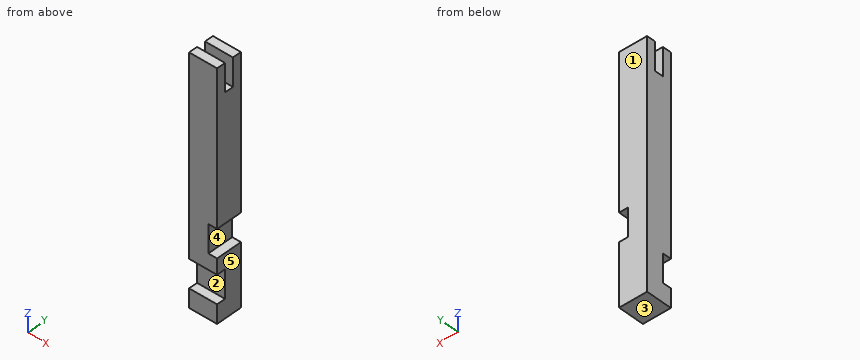
from build123d import *

# Parameters (mm, degrees)
F0_W     = 114.3
F0_H     = 106.68
F1_DEPTH = 990.6
F2_W     = 114.3
F2_H     = 35.56
F3_DEPTH = 114.3
F4_W     = 114.3
F4_H     = 114.3
F5_DEPTH = 35.56
F6_W     = 106.68
F6_H     = 114.3
F7_DEPTH = 35.56


with BuildPart() as f1:
    # F0 (on Top) → F1 (new body)
    with BuildSketch(Plane.XY):
        Rectangle(F0_W, F0_H)
    extrude(amount=F1_DEPTH)

    # F2 (on face) → F3 (cut)
    with BuildSketch(Plane.XY.offset(990.6)):
        Rectangle(F2_W, F2_H)
    extrude(amount=-F3_DEPTH, mode=Mode.SUBTRACT)

    # F4 (on face) → F5 (cut)
    with BuildSketch(Plane.XZ.offset(53.34)):
        with Locations((0, 133.35)):
            Rectangle(F4_W, F4_H)
    extrude(amount=-F5_DEPTH, mode=Mode.SUBTRACT)

    # F6 (on face) → F7 (cut)
    with BuildSketch(Plane.YZ.offset(57.15)):
        with Locations((0, 311.15)):
            Rectangle(F6_W, F6_H)
    extrude(amount=-F7_DEPTH, mode=Mode.SUBTRACT)


solid = f1.part
Check sheet for the modelled part. Datum: model origin and axes. Units: mm. Face numbers are marked on the shaded views. A direction names the side the tool comes from. Round coordinates to 2 decimals unless told otherwise and drop trailing zeros. Order: outer loops, then holes, each group sorted by start corner. A loop starts at its lowest first (then second) coordinate and runs counter-clockwise, first axis right, second up.
(1) Draft check along Z on the marked faces 3, 4 and 5. Enter one of: pulls with the +Z half, pulls with the -Z half, needs draft (parallel to the pull), parting line crosses it, or undercut.
(2) Access from +Z, -Z, +X, -X, +Y, -Y to the whole of each face (thin tool, end or side, straight path). Record for the marked faces 1 and 2.
(3) Cross-section at B-B, the plane y = -37.5. Enter the section's corners in (x, z), and give its area (3 significant figures).
(4) Cross-section at A-A, the plane z = 912. Enter the section's corners in (x, y), and give its area (3 significant figures).
(5) Cross-section at C-C, the plane y = 8. Enter the section's corners in (x, z).
(6) Cross-section at D-D, the plane x = 0. Enter the section's corners in (y, z), and give its area (3 significant figures).
(7) Scan lines: probe 1 along Z at (x, y) = (47, -44); probe 2 along Z at (x, y) = (48, -11.5); probe 3 along Z at (x, y) = (-51, -26). Record each from-to range of solid material in increasing order.
(8) Go/stop test with flat-tipped pins: P1, Ø12, axis at x = -39, y = 14.5, coming from the -Z side; P2, Ø18, axis at x = 24.5, y = 2.5, coming from the +Z side. Record where each tip stops, or that it passes through.
Check sheet entries:
1. face 3: pulls with the -Z half
1. face 4: undercut
1. face 5: needs draft
2. face 1: +Z, -Z, +X, -X, +Y
2. face 2: +X, -X, -Y
3. outline: (-57.15, 0) - (57.15, 0) - (57.15, 76.2) - (-57.15, 76.2) - close; (-57.15, 190.5) - (57.15, 190.5) - (57.15, 254) - (21.59, 254) - (21.59, 368.3) - (57.15, 368.3) - (57.15, 990.6) - (-57.15, 990.6) - close
3. area: 96,100 mm2
4. outline: (-57.15, -53.34) - (57.15, -53.34) - (57.15, -17.78) - (-57.15, -17.78) - close; (-57.15, 17.78) - (57.15, 17.78) - (57.15, 53.34) - (-57.15, 53.34) - close
4. area: 8,130 mm2
5. outline: (-57.15, 0) - (57.15, 0) - (57.15, 254) - (21.59, 254) - (21.59, 368.3) - (57.15, 368.3) - (57.15, 876.3) - (-57.15, 876.3) - close
6. outline: (-53.34, 0) - (53.34, 0) - (53.34, 990.6) - (17.78, 990.6) - (17.78, 876.3) - (-17.78, 876.3) - (-17.78, 990.6) - (-53.34, 990.6) - (-53.34, 190.5) - (-17.78, 190.5) - (-17.78, 76.2) - (-53.34, 76.2) - close
6. area: 97,500 mm2
7. probe 1: z = 0 to 76.2, 190.5 to 254, 368.3 to 990.6
7. probe 2: z = 0 to 254, 368.3 to 876.3
7. probe 3: z = 0 to 76.2, 190.5 to 990.6
8. P1: stops at z = 0
8. P2: stops at z = 876.3
